Geometry: final body of the model. Coordinates: model frame, mm. Face numbers are marked on the shaded views. A direction names the side the tool comes from. Round coordinates to 2 decimals unless told otherwise and drop trailing zeros. Order: outer loops, then holes, each group sorted by start corner. A loop starts at its lowest first (then second) coordinate and runs counter-clockwise, first axis right, second up. Notation, with made-up numbers: M 5,-1.75 L 12,-1.75 A11 ccw 12,10.25 Z; hole C 49.25,26 d4. An arc over 180 degrees is marked long. Return JSON: item names as keys, results as strings. Group by question number.
Q1. Contact query for flat-ended pins moving along their axis: pin 1 (4.5 mm diameter, centred on x = 4.5, z = -4, fed in from +Y); pin 2 (4 mm diameter, centred on y = 3, z = 1, fed in from +X); pin 3 (3 mm diameter, centred on x = 27.5, z = 16, fed in from -Y); pin 4 (1 mm diameter, centred on x = -1.5, z = 66.5, fed in from -Y). Output: stop coordinate, or through.
Q2. Cut plane D-D on y = 45. Output: boundary loops of the cut face in (x, z), and give its area (3 significant figures).
Q3. Cut plane B-B on y = -45. Output: boundary loops of the cut face in (x, z), and give its area (3 significant figures).
Q4. Ray query, probe 1 along Y at (x, z) = (-25, -3.25); probe 2 along Y at (x, z) = (25, -10.5); probe 3 along X at (y, z) = (6, 11.5). Return the intervals inside material, ascending.
Q5. Access query for the marked faces 1, 2 and 3. Directions: +Z, -Z, +X, -X, +Y, -Y. A direction counts if a zero-diameter tool reaches every point of the face in a straight line with its end or side. Return the directions, or none.
Q6. Cut plane C-C on x = 15. Output: boundary loops of the cut face in (y, z).
Q7. Cut plane A-A on x = -25. Output: boundary loops of the cut face in (y, z).
Q8. Mould query, pull axis Y, two halves, no side actions, for the marked faces 4, 5 and 6. Classes: released by +Y, released by -Y, zero draft, split by the parting line, or undercut.
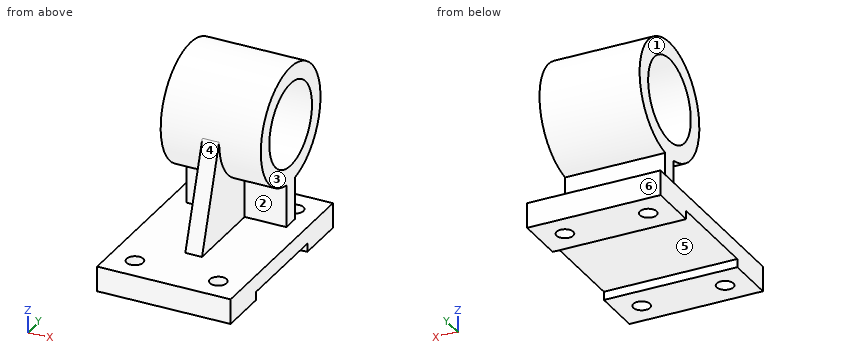
Solid Edge part; units mm, degrees
sketch "Sketch1" plane through (0, 0, 0) normal (1, 0, 0) x (0, 1, 0)
  line L0 (-60, 0) -> (60, 0)
  line L1 (60, -15) -> (60, 0)
  line L2 (30, -15) -> (60, -15)
  line L3 (30, -10) -> (30, -15)
  line L4 (-30, -10) -> (30, -10)
  line L5 (-30, -15) -> (-30, -10)
  line L6 (-60, -15) -> (-30, -15)
  line L7 (-60, 0) -> (-60, -15)
extrude "Protrusion1" add sketch "Sketch1" along normal mid plane 80
sketch "Sketch2" plane through (0, 0, 0) normal (1, 0, 0) x (0, 1, 0)
  line L0 (35, 0) -> (35, 25.359)
  line L1 (25, 25.359) -> (25, 0)
  line L2 (25, 0) -> (35, 0)
  arc A0 (25, 25.359) -> (35, 25.359) centre (30, 60) cw
  circle A1 centre (30, 60) radius 25
extrude "ExtrudedProtrusion_2" add sketch "Sketch2" along normal mid plane 60
sketch "Sketch3" plane through (0, 0, 0) normal (1, 0, 0) x (0, 1, 0)
  line L0 (-25, 0) -> (-5, 60)
  line L1 (25, 0) -> (-25, 0)
  line L2 (25, 25.359) -> (25, 0)
  arc A0 (-5, 60) -> (25, 25.359) centre (30, 60) ccw
extrude "ExtrudedProtrusion_3" add sketch "Sketch3" along normal mid plane 10
sketch "Sketch4" plane through (0, 0, 0) normal (0, 0, 1) x (1, 0, 0)
  circle A0 centre (25, -45) radius 5
  circle A1 centre (-25, -45) radius 5
  circle A2 centre (25, 45) radius 5
  circle A3 centre (-25, 45) radius 5
extrude "ExtrudedCutout_1" cut sketch "Sketch4" against normal blind 57.0095
Result sheet:
{
 "1": {"pin 1": "stops at y = 60", "pin 2": "stops at x = 40", "pin 3": "stops at y = 25", "pin 4": "stops at y = -4.48"},
 "2": {"outline": "M -40,-15 L -30,-15 L -30,0 L -40,0 Z; M -30,28.38 L 30,28.38 L 30,40 L -30,40 Z; M -30,80 L 30,80 L 30,91.62 L -30,91.62 Z; M -20,-15 L 20,-15 L 20,0 L -20,0 Z; M 30,-15 L 40,-15 L 40,0 L 30,0 Z", "area": "2,290 mm²"},
 "3": {"outline": "M -40,-15 L -30,-15 L -30,0 L -40,0 Z; M -20,-15 L 20,-15 L 20,0 L -20,0 Z; M 30,-15 L 40,-15 L 40,0 L 30,0 Z", "area": "900 mm²"},
 "4": {"probe 1": "y = -60 to -50, -40 to 40, 50 to 60", "probe 2": "y = -60 to -50, -40 to -30, 30 to 40, 50 to 60", "probe 3": "x = -5 to 5"},
 "5": {"face 1": "+Z, -X, +Y, -Y", "face 2": "+X, -Y", "face 3": "+Z, +X, +Y, -Y"},
 "6": {"outline": "M -60,-15 L -30,-15 L -30,-10 L 30,-10 L 30,-15 L 60,-15 L 60,0 L 35,0 L 35,25.36 A35 ccw long 25,25.36 L 25,0 L -60,0 Z; hole C 30,60 d50"},
 "7": {"outline": "M -60,-15 L -50,-15 L -50,0 L -60,0 Z; M -40,-15 L -30,-15 L -30,-10 L 30,-10 L 30,-15 L 40,-15 L 40,0 L 35,0 L 35,25.36 A35 ccw long 25,25.36 L 25,0 L -40,0 Z; M 50,-15 L 60,-15 L 60,0 L 50,0 Z; hole C 30,60 d50"},
 "8": {"face 4": "released by -Y", "face 5": "undercut", "face 6": "released by +Y"}
}
